CAD build for the part. Positions are in the model's coordinates, mm. Face numbers are marked on the shaded views. A direction names the side the tool comes from. Coordinates: 2 decimals unless noted, no trailing zeros. Order: outer loops, then holes, each group sorted by start corner. A loop starts at its lowest first (then second) coordinate and runs counter-clockwise, first axis right, second up. Notation, with made-up numbers: M 80,80 L 114,80 A20 ccw 114,114 Z; hole C 67,83.25 d5. An arc over 180 degrees is marked long. One line per item, written item: value.
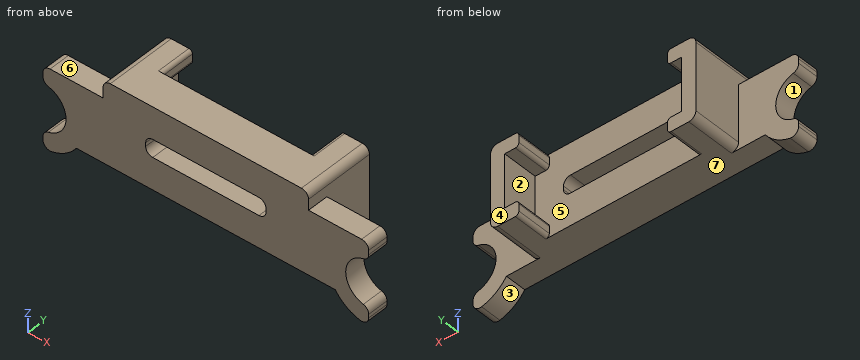
from build123d import *

# Parameters (mm, degrees)
MAIN_BODY_DEPTH            = 3
SKETCH2_W                  = 29
SKETCH2_H                  = 11.5
FAN_OFFSET_DEPTH           = 2
FAN_FRAME_DEPTH            = 5
SKETCH4_W                  = 17
SKETCH4_H                  = 2.5
SPEED_HOLE_DEPTH           = 6
CONTOURING_R               = 1
FIT_CLEARANCE_CONTOURING_R = 0.5


with BuildPart() as part:
    # Sketch1 → Main Body (new body)
    with BuildSketch(Plane(origin=(0, 0, 0), x_dir=(1, 0, 0), z_dir=(0, 1, 0))):
        with BuildLine():
            Line((-23, -3.25), (-23, -5.73))
            Line((-23, -5.73), (-14.5, -5.73))
            Line((-14.5, -5.73), (-14.5, -8.25))
            Line((-14.5, -8.25), (14.5, -8.25))
            Line((14.5, -8.25), (14.5, -5.73))
            Line((14.5, -5.73), (23, -5.73))
            Line((23, -5.73), (23, -3.25))
            ThreePointArc((23, -3.25), (19.75, 0), (23, 3.25))
            Line((23, 3.25), (23, 5.73))
            ThreePointArc((23, 5.73), (20.334441897, 5.072248022), (18.280847534, 3.25))
            Line((18.280847534, 3.25), (-18.280847534, 3.25))
            ThreePointArc((-18.280847534, 3.25), (-20.334441897, 5.072248022), (-23, 5.73))
            Line((-23, 5.73), (-23, 3.25))
            ThreePointArc((-23, 3.25), (-19.75, 0), (-23, -3.25))
        make_face()
    extrude(amount=MAIN_BODY_DEPTH)

    # Sketch2 → Fan Offset (add)
    with BuildSketch(Plane(origin=(0, 3, 0), x_dir=(1, 0, 0), z_dir=(0, 1, 0))):
        with Locations((0, -2.5)):
            Rectangle(SKETCH2_W, SKETCH2_H)
    extrude(amount=FAN_OFFSET_DEPTH)

    # Sketch3 → Fan Frame (add)
    with BuildSketch(Plane(origin=(0, 5, 0), x_dir=(1, 0, 0), z_dir=(0, 1, 0))):
        Polygon((-10.5, 3.25), (-14.5, 3.25), (-14.5, -8.25), (-10.5, -8.25), (-10.5, -6.25), (-12.5, -6.25), (-12.5, 1.25), (-10.5, 1.25), align=None)
        Polygon((12.5, -6.25), (12.5, 1.25), (10.5, 1.25), (10.5, 3.25), (14.5, 3.25), (14.5, -8.25), (10.5, -8.25), (10.5, -6.25), align=None)
    extrude(amount=FAN_FRAME_DEPTH)

    # Sketch4 → Speed Hole (cut, through all)
    with BuildSketch(Plane(origin=(0, 5, 0), x_dir=(1, 0, 0), z_dir=(0, 1, 0))):
        with Locations((0, -2.5)):
            Rectangle(SKETCH4_W, SKETCH4_H)
    extrude(amount=-SPEED_HOLE_DEPTH, mode=Mode.SUBTRACT)

    # Contouring
    contouring_edges = [part.edges().sort_by_distance(p)[0] for p in [
        (-14.5, 6.5, -3.25),
        (14.5, 6.5, -3.25),
        (14.5, 5, 8.25),
        (-14.5, 5, 8.25),
        (23, 1.5, 5.73),
        (23, 1.5, 3.25),
        (23, 1.5, -3.25),
        (23, 1.5, -5.73),
        (-23, 1.5, 5.73),
        (-23, 1.5, 3.25),
        (-23, 1.5, -3.25),
        (-23, 1.5, -5.73),
        (-8.5, 2.5, 1.25),
        (-8.5, 2.5, 3.75),
        (8.5, 2.5, 3.75),
        (8.5, 2.5, 1.25),
    ]]
    fillet(contouring_edges, radius=CONTOURING_R)

    # Fit Clearance - Contouring
    fit_clearance_contouring_edges = [part.edges().sort_by_distance(p)[0] for p in [
        (10.5, 7.5, -3.25),
        (-10.5, 7.5, -3.25),
        (-10.5, 7.5, 8.25),
        (-10.5, 7.5, 6.25),
        (10.5, 7.5, 8.25),
        (10.5, 7.5, 6.25),
        (10.5, 7.5, -1.25),
        (-10.5, 7.5, -1.25),
    ]]
    fillet(fit_clearance_contouring_edges, radius=FIT_CLEARANCE_CONTOURING_R)


solid = part.part
Q1. Slice it at C-C (y = 6). List the corners of the cut face in (x, z), plus the area to 3 significant figures.
Recorded:
outline: M -14.5,-2.25 A1 ccw -13.5,-3.25 L -11,-3.25 A0.5 ccw -10.5,-2.75 L -10.5,-1.75 A0.5 ccw -11,-1.25 L -12.5,-1.25 L -12.5,6.25 L -11,6.25 A0.5 ccw -10.5,6.75 L -10.5,7.75 A0.5 ccw -11,8.25 L -13.5,8.25 A1 ccw -14.5,7.25 Z; M 10.5,-2.75 A0.5 ccw 11,-3.25 L 13.5,-3.25 A1 ccw 14.5,-2.25 L 14.5,7.25 A1 ccw 13.5,8.25 L 11,8.25 A0.5 ccw 10.5,7.75 L 10.5,6.75 A0.5 ccw 11,6.25 L 12.5,6.25 L 12.5,-1.25 L 11,-1.25 A0.5 ccw 10.5,-1.75 Z
area: 60.7 mm^2
Q2. Mould opens along Z. For the marked faces 1, 2, 3 and 4 say: released by +Z, released by -Z, zero draft, split by the parting line, or undercut.
Recorded:
face 1: undercut
face 2: undercut
face 3: released by -Z
face 4: zero draft
Q3. Drill centre lines: line 1 along Z through (x, y) = (3, 2.25); line 2 along X through (y, z) = (8, 4.25); line 3 along Y through (x, z) = (2.5, 4.5). Where is each one in solid material? Low to high.
Recorded:
line 1: z = -3.25 to 1.25, 3.75 to 8.25
line 2: x = -14.5 to -12.5, 12.5 to 14.5
line 3: y = 0 to 5
Q4. Pin check, flat tips, straight feed: pin 1 Ø1 at (x, z) = (-13.5, 3.5) entering from -Y; pin 2 Ø1.1 at (y, z) = (7.5, 7.5) entering from +X; pin 3 Ø0.6 at (y, z) = (3, 2.5) entering from +X; pin 4 Ø0.9 at (x, y) = (-19.5, 1) entering from +Z. Stop position of each tip, or through.
Recorded:
pin 1: stops at y = 0
pin 2: stops at x = 14.5
pin 3: stops at x = 21.35
pin 4: stops at z = 5.73
Q5. Slice it at A-A (x = 6). List the corners of the cut face in (y, z), plus the area to 3 significant figures.
Recorded:
outline: M 0,-3.25 L 5,-3.25 L 5,1.25 L 0,1.25 Z; M 0,3.75 L 5,3.75 L 5,8.25 L 0,8.25 Z
area: 45.0 mm^2
Q6. Slice it at D-D (z = 0). List the corners of the cut face in (x, y).
Recorded:
outline: M -19.75,0 L 19.75,0 L 19.75,3 L 14.5,3 L 14.5,10 L 12.5,10 L 12.5,5 L -12.5,5 L -12.5,10 L -14.5,10 L -14.5,3 L -19.75,3 Z
Q7. Which spindle directions (+Z, -Z, +X, -X, +Y, -Y) get a long thin tool onto all of the face, cutting with end or side? Do the marked faces 5, 6 and 7. Say none if no direction does.
Recorded:
face 5: +Y
face 6: +Z, -X, +Y, -Y
face 7: -Z, +Y, -Y
